Geometry check sheet. Reference: drawing and pictorial views, mm from the part's lowest x, y, z. A direction names the side the tool comes from. Round coordinates to 2 decimals unless told otherwise and drop trailing zeros. Order: outer loops, then holes, each group sorted by start corner. A loop starts at its lowest first (then second) coordinate and runs counter-clockwise, first axis right, second up. Notation, with made-up numbers: (-10, -30) -> (47, -30) arc R29 cw to (47, -8) -> close; hole circle Ø4 at (27, 46). An arc over 180 degrees is marked (long way). Return JSON: item names as keys, results as strings. Group by question number.
1) Section check B-B on y = 11.25. State how many separate pieces and enclosed holes the cut face has.
2) Section check C-C on y = 8.75. Enter the section's corners in (x, z), plus the area to 3 significant figures.
3) Section check A-A on y = 4.5. Enter the section's corners in (x, z).
4) Tool access check on the marked faces 1 and 2. Record the directions out of +Z, -Z, +X, -X, +Y, -Y that give a thin tool (end or side, any length) a straight path to the whole face; none if there is none.
5) Scan lines: L1, parallel to X at y = 10.75, z = 2.85 (1 decimal); L2, parallel to Y at x = 2.4, z = 0.35; L3, parallel to Y at x = 3.3, z = 3.1. Record each from-to range of solid material in increasing order.
6) Depth check by flat-ended pin: pin 1 (2 mm diameter, centred on x = 3.5, y = 8, fed in from -Z); pin 2 (1 mm diameter, centred on x = 2, z = 4.5, fed in from -Y); pin 3 (1.8 mm diameter, centred on x = 3, z = 4, fed in from +Y); pin 4 (3 mm diameter, centred on x = 1, z = 4.5, fed in from -Y). Enter the tip coordinate at first touch or a pass-through.
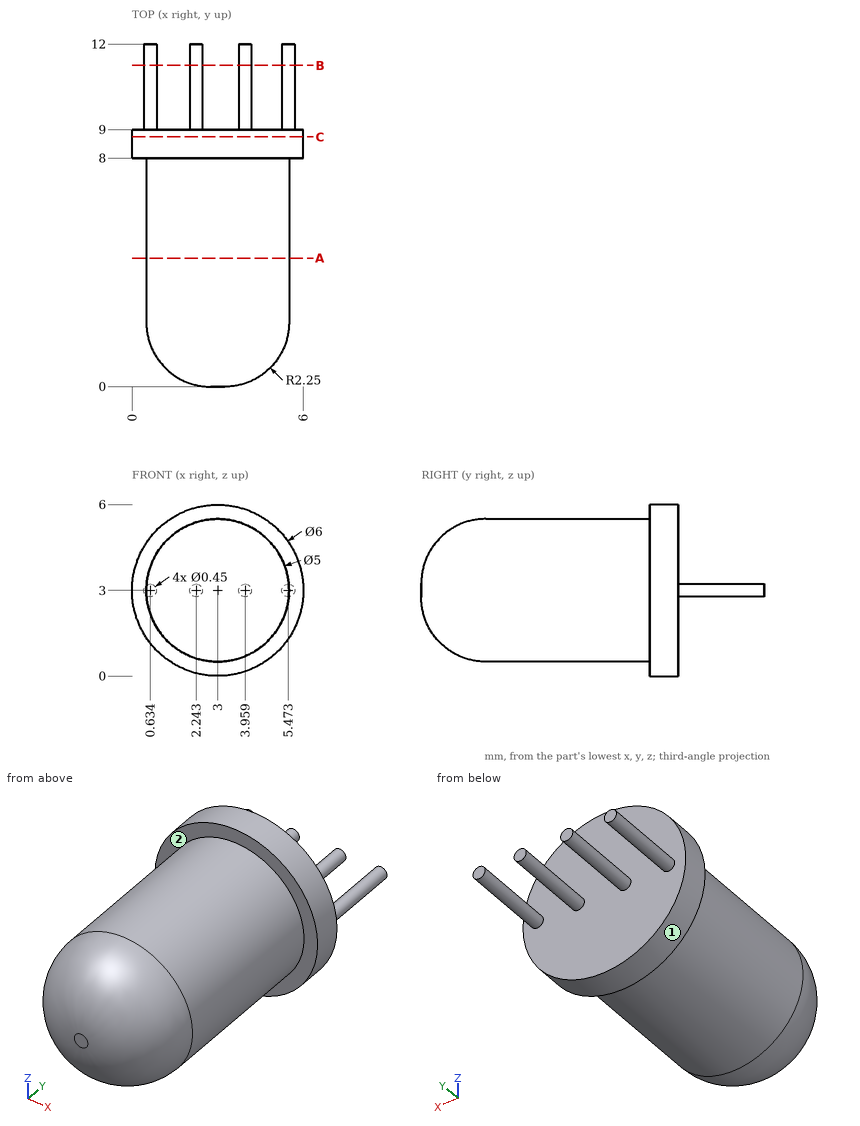
Check result:
{
 "1": {"separate pieces": "4", "enclosed holes": "0"},
 "2": {"outline": "circle Ø6 at (3, 3)", "area": "28.3 mm^2"},
 "3": {"outline": "circle Ø5 at (3, 3)"},
 "4": {"face 1": "+Y, -Y", "face 2": "-Y"},
 "5": {"L1": "0.5 to 0.8, 2.1 to 2.4, 3.8 to 4.1, 5.3 to 5.6", "L2": "8 to 9", "L3": "0 to 9"},
 "6": {"pin 1": "z = 0", "pin 2": "y = 0.26", "pin 3": "y = 9", "pin 4": "y = 0.13"}
}
